Check sheet for the modelled part. Datum: model origin and axes. Units: mm. Face numbers are marked on the shaded views. Round coordinates to 2 decimals unless told otherwise and drop trailing zeros. Order: outer loops, then holes, each group sorted by start corner. A loop starts at its lowest first (then second) coordinate and runs counter-clockwise, first axis right, second up. Notation, with made-up numbers: (27.25, -0.75) -> (31.25, -0.75) arc R23 cw to (31.25, 13.25) -> close; hole circle Ø9 at (59, -25). An arc over 180 degrees is marked (long way). Answer in a Markdown table with one row per item.
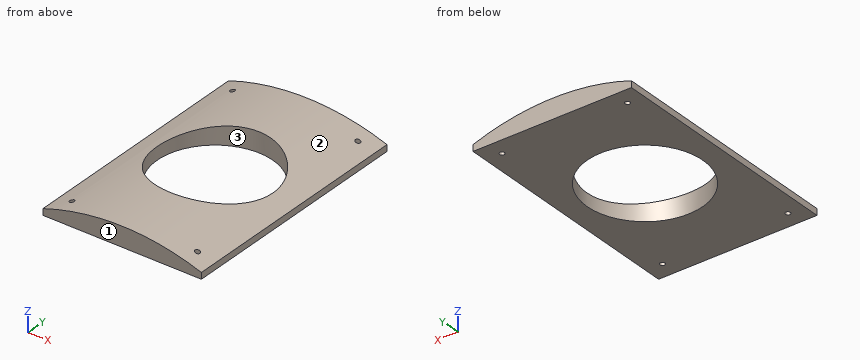
from build123d import *

# Parameters (mm, degrees)
PAD008_DEPTH    = 147
SKETCH029_R     = 35
POCKET004_DEPTH = 12.001
SKETCH049_R     = 1.5
POCKET013_DEPTH = 12.001


with BuildPart() as part:
    # Sketch028 → Pad008 (new body)
    with BuildSketch(Plane.XZ):
        with BuildLine():
            Line((-327.151421, 0), (-231.151421, 0))
            Line((-231.151421, 0), (-231.151421, 3.854468))
            ThreePointArc((-231.151421, 3.854468), (-279.151421, 12), (-327.151421, 3.854468))
            Line((-327.151421, 0), (-327.151421, 3.854468))
        make_face()
    extrude(amount=PAD008_DEPTH)

    # Sketch029 (on DatumPlane) → Pocket004 (cut, through all)
    with BuildSketch(Plane(origin=(0, 0, 0), x_dir=(1, 0, 0), z_dir=(0, 0, -1))):
        with Locations((-279.151421, 73.5)):
            Circle(SKETCH029_R)
    extrude(amount=-POCKET004_DEPTH, mode=Mode.SUBTRACT)

    # Sketch049 (on Face1 of Pocket004) → Pocket013 (cut, through all)
    with BuildSketch(Plane(origin=(0, 0, 0), x_dir=(1, 0, 0), z_dir=(0, 0, -1))):
        with Locations((-317.151421, 137)):
            Circle(SKETCH049_R)
        with Locations((-241.151421, 137)):
            Circle(SKETCH049_R)
        with Locations((-317.151421, 10)):
            Circle(SKETCH049_R)
        with Locations((-241.151421, 10)):
            Circle(SKETCH049_R)
    extrude(amount=-POCKET013_DEPTH, mode=Mode.SUBTRACT)


with BuildPart() as part_1:
    # Body006 placement: moved
    add(part.part.moved(Location((436.71651, -6.430456, -3.949142))))


solid = part_1.part
Item 1: Mould release check, pull along X, two halves, no side actions. Record for the marked faces 1, 2 and 3: pulls with the +X half, pulls with the -X half, needs draft (parallel to the pull), parting line crosses it, or undercut.
Result sheet:
| item | result |
|---|---|
| face 1 | needs draft |
| face 2 | parting line crosses it |
| face 3 | undercut |
Item 2: Depth check by flat-ended pin: P1, Ø4, axis at x = 119.57, y = -143.43, coming from the +Z side; P2, Ø12, axis at x = 154.5, y = -137, coming from the +Z side; P3, Ø5, axis at x = 119.57, y = -16.43, coming from the -Z side. Enter the tip coordinate at first touch or a pass-through.
Result sheet:
| item | result |
|---|---|
| P1 | stops at z = 3.53 |
| P2 | stops at z = 8.05 |
| P3 | stops at z = -3.95 |
Item 3: Cross-section at C-C (x = 161). Record the boundary of the cut face in (y, z).
Result sheet:
| item | result |
|---|---|
| outline | (-153.43, -3.95) -> (-114.76, -3.95) -> (-114.76, 8.01) -> (-153.43, 8.01) -> close; (-45.1, -3.95) -> (-6.43, -3.95) -> (-6.43, 8.01) -> (-45.1, 8.01) -> close |
Item 4: Cross-section at B-B (z = -2). Record the boundary of the cut face in (x, y).
Result sheet:
| item | result |
|---|---|
| outline | (109.57, -153.43) -> (205.57, -153.43) -> (205.57, -6.43) -> (109.57, -6.43) -> close; hole circle Ø3 at (119.57, -143.43); hole circle Ø3 at (119.57, -16.43); hole circle Ø70 at (157.57, -79.93); hole circle Ø3 at (195.57, -143.43); hole circle Ø3 at (195.57, -16.43) |
Item 5: Cross-section at A-A (y = -77.5). Record the boundary of the cut face in (x, z), and give its area (3 significant figures).
Result sheet:
| item | result |
|---|---|
| outline | (109.57, -3.95) -> (122.65, -3.95) -> (122.65, 3.8) arc R145.5 ccw to (109.57, -0.09) -> close; (192.48, -3.95) -> (205.57, -3.95) -> (205.57, -0.09) arc R145.5 ccw to (192.48, 3.8) -> close |
| area | 155 mm^2 |
Item 6: Cross-section at D-D (y = -127.5). Record the boundary of the cut face in (x, z).
Result sheet:
| item | result |
|---|---|
| outline | (109.57, -3.95) -> (205.57, -3.95) -> (205.57, -0.09) arc R145.5 ccw to (109.57, -0.09) -> close |
Item 7: Scan lines: line 1 (X direction, y = -143.5, z = -1); line 2 (Y direction, x = 143, z = 7); line 3 (Y direction, x = 184.5, z = -2.25). Record each from-to range of solid material in increasing order. Write a range as [from, to].
Result sheet:
| item | result |
|---|---|
| line 1 | x = [109.57, 118.07], [121.06, 194.07], [197.06, 205.57] |
| line 2 | y = [-153.43, -111.76], [-48.11, -6.43] |
| line 3 | y = [-153.43, -102.28], [-57.58, -6.43] |
